from build123d import *

# Parameters (mm, degrees)
BOSS_EXTRUDE1_DEPTH = 6
SKETCH2_W           = 30
SKETCH2_H           = 14
SKETCH2_W_2         = 97
SKETCH2_H_2         = 40
SKETCH2_W_3         = 47
SKETCH2_H_3         = 57
CUT_EXTRUDE1_DEPTH  = 6


with BuildPart() as part:
    # Model → Boss-Extrude1 (new body)
    with BuildSketch(Plane.XY):
        Polygon((221, 430), (221, 414), (215, 414), (215, 402), (221, 402), (221, 390), (215, 390), (215, 378), (221, 378), (221, 366), (215, 366), (215, 354), (221, 354), (221, 342), (215, 342), (215, 330), (221, 330), (221, 318), (215, 318), (215, 306), (221, 306), (221, 294), (215, 294), (215, 282), (221, 282), (221, 270), (215, 270), (215, 258), (221, 258), (221, 246), (215, 246), (215, 234), (221, 234), (221, 218), (237, 218), (237, 224), (249, 224), (249, 218), (261, 218), (261, 224), (273, 224), (273, 218), (285, 218), (285, 224), (297, 224), (297, 218), (309, 218), (309, 224), (321, 224), (321, 218), (333, 218), (333, 224), (345, 224), (345, 218), (357, 218), (357, 224), (369, 224), (369, 218), (381, 218), (381, 224), (393, 224), (393, 218), (405, 218), (405, 224), (417, 224), (417, 218), (429, 218), (429, 224), (441, 224), (441, 218), (453, 218), (453, 224), (465, 224), (465, 218), (477, 218), (481, 218), (481, 234), (487, 234), (487, 246), (481, 246), (481, 258), (487, 258), (487, 270), (481, 270), (481, 282), (487, 282), (487, 294), (481, 294), (481, 306), (487, 306), (487, 318), (481, 318), (481, 330), (487, 330), (487, 342), (481, 342), (481, 354), (487, 354), (487, 366), (481, 366), (481, 378), (487, 378), (487, 390), (481, 390), (481, 402), (487, 402), (487, 414), (481, 414), (481, 430), (465, 430), (465, 424), (453, 424), (453, 430), (441, 430), (441, 424), (429, 424), (429, 430), (417, 430), (417, 424), (405, 424), (405, 430), (393, 430), (393, 424), (381, 424), (381, 430), (369, 430), (369, 424), (357, 424), (357, 430), (345, 430), (345, 424), (333, 424), (333, 430), (321, 430), (321, 424), (309, 424), (309, 430), (297, 430), (297, 424), (285, 424), (285, 430), (273, 430), (273, 424), (261, 424), (261, 430), (249, 430), (249, 424), (237, 424), (237, 430), (225, 430), align=None)
    extrude(amount=BOSS_EXTRUDE1_DEPTH)

    # Sketch2 → Cut-Extrude1 (cut)
    with BuildSketch(Plane.XY.offset(6)):
        with Locations((351, 395)):
            Rectangle(SKETCH2_W, SKETCH2_H)
        with Locations((351, 346)):
            Rectangle(SKETCH2_W_2, SKETCH2_H_2)
        with Locations((351, 277.5)):
            Rectangle(SKETCH2_W_3, SKETCH2_H_3)
    extrude(amount=-CUT_EXTRUDE1_DEPTH, mode=Mode.SUBTRACT)


solid = part.part
Read the model definition and answer for the solid it produces. Units are mm, in the model's axes. A direction names the side the tool comes from. Give positions to 0.01 mm unless a question says otherwise; leave off trailing zeros. Loops run counter-clockwise (first coordinate to the right, second up) from the corner with the lowest first, then second, coordinate; pieces in that order, holes last. Notation, with made-up numbers: (-37.75, -35) - (11.25, -35) arc R21 cw to (11.25, -9) - close; hole circle Ø10 at (15, -37). An arc over 180 degrees is marked (long way). Answer as CSV lines item,"result". Start each with the question number.
1) Find section D-D (x = 270). Write down the section's boundary in (y, z).
2) Find section C-C (y = 334). Write down the section's boundary in (x, z), then the cut area to 3 significant figures.
3) Straight lines are drawn through the part: L1, parallel to Y at x = 373, z = 3.45; L2, parallel to Y at x = 396.5, z = 5.7; L3, parallel to X at y = 355, z = 2.8. For each, find the intervals that lie inside material, in ascending order. Write a range as from..to.
4) Find section A-A (y = 279). Write down the section's boundary in (x, z).
5) Each of these flat-tipped pins is pushed along its axis until it touches: pin 1 Ø3 at (x, z) = (484.5, 1.5) entering from -Y; pin 2 Ø3 at (y, z) = (249.5, 4) entering from +X; pin 3 Ø1.8 at (x, z) = (268, 2) entering from -Y. Where does it stop, or does it pass through?
6) Which of the six approach directions +Z, -Z, +X, -X, +Y, -Y give full straight-line access (tool end or side, diameter ignored) to faces 4 (the face through (484, 378, 3)), 5 (the face through (459, 424, 3)), 6 (the face through (221, 372, 3))?
7) Determine the mould class of faces 1 (the face through (215, 264, 3)), 2 (the face through (487, 264, 3)), 3 (the face through (435, 424, 3)) for opening direction X: released by +X, released by -X, zero draft, split by the parting line, or undercut.
8) Find section B-B (z = 4.2). State how many separate pieces and enclosed holes the cut face has, then the cut area to 3 significant figures.
Findings below:
1,outline,"(224, 0) - (424, 0) - (424, 6) - (224, 6) - close"
2,outline,"(215, 0) - (302.5, 0) - (302.5, 6) - (215, 6) - close; (399.5, 0) - (487, 0) - (487, 6) - (399.5, 6) - close"
2,area,"1,050 mm^2"
3,L1,"218..249, 306..326, 366..430"
3,L2,"218..326, 366..430"
3,L3,"215..302.5, 399.5..487"
4,outline,"(221, 0) - (327.5, 0) - (327.5, 6) - (221, 6) - close; (374.5, 0) - (481, 0) - (481, 6) - (374.5, 6) - close"
5,pin 1,"y = 234"
5,pin 2,"x = 481"
5,pin 3,"y = 224"
6,face 4,"+Z, -Z, +X"
6,face 5,"+Z, -Z, +Y"
6,face 6,"+Z, -Z, -X"
7,face 1,"released by -X"
7,face 2,"released by +X"
7,face 3,"undercut"
8,separate pieces,"1"
8,enclosed holes,"3"
8,area,"47,900 mm^2"
